```python
from build123d import *

# Parameters (mm, degrees)
SKETCH_1_R      = 50
SKETCH_1_R_2    = 40
EXTRUDE_1_DEPTH = 85
CHAMFER_1_SIZE  = 1
M10X1_0_1_D     = 9
M10X1_0_1_DEPTH = 25
M10X1_0_1_TIP   = 2.703872786


with BuildPart() as part:
    # 草图1 → 凸台-拉伸1 (new body)
    with BuildSketch(Plane(origin=(0, 0, 0), x_dir=(0, 0, -1), z_dir=(1, 0, 0))):
        Circle(SKETCH_1_R)
        Circle(SKETCH_1_R_2, mode=Mode.SUBTRACT)
    extrude(amount=EXTRUDE_1_DEPTH)

    # 倒角1
    chamfer_1_edges = [part.edges().sort_by_distance(p)[0] for p in [
        (0, 0, 50),
        (85, 0, 50),
        (0, 0, 40),
        (85, 0, 40),
    ]]
    chamfer(chamfer_1_edges, length=CHAMFER_1_SIZE)

    # M10x1.0 螺纹孔1
    with Locations(Plane(origin=(0, 50, 0), x_dir=(1, 0, 0), z_dir=(0, 1, 0))):
        with Locations((70, 0)):
            Hole(M10X1_0_1_D / 2, depth=M10X1_0_1_DEPTH)
            with Locations((0, 0, -(M10X1_0_1_DEPTH + M10X1_0_1_TIP / 2))):  # 118° drill point
                Cone(0, M10X1_0_1_D / 2, M10X1_0_1_TIP, mode=Mode.SUBTRACT)


solid = part.part
```
Could you check a few things on this model? Use its own coordinates, in mm. Coordinates: 2 decimals unless noted, no trailing zeros. Write each loop counter-clockwise with the first axis right and the second up, starting at its lowest first coordinate (ties: lowest second). Pieces come first, ordered by that corner, then holes. Notation, with made-up numbers: (64, 1) - (95, 1) arc R22 cw to (95, 15) - close; hole circle Ø6 at (38.25, 34.25). An arc over 180 degrees is marked (long way). Use a Markdown table: item, result.
Q1. Thinking about a two-plate mould opening in X: for faces 1 (the cylindrical face through (65.84, 44.8, 1.72)), 2 (the flat face through (85, -40, 11)), 3 (the flat face through (0, -40, 11)), which applies, +X half, -X half, draft (parallel to the pull), parting line (faces both ways), or undercut?
Geometry check:
| item | result |
|---|---|
| face 1 | undercut |
| face 2 | +X half |
| face 3 | -X half |
Q2. Imagine slicing it at A-A (z = 0). List the corners of the cut face in (x, y) for me.
Geometry check:
| item | result |
|---|---|
| outline | (0, -49) - (1, -50) - (84, -50) - (85, -49) - (85, -41) - (84, -40) - (1, -40) - (0, -41) - close; (0, 41) - (1, 40) - (65.5, 40) - (65.5, 50) - (1, 50) - (0, 49) - close; (74.5, 40) - (84, 40) - (85, 41) - (85, 49) - (84, 50) - (74.5, 50) - close |
Q3. I'm going to push flat-ended pins straight in: pin 1 Ø4 at (x, z) = (50, -2) entering from -Y; pin 2 Ø5 at (y, z) = (-7.5, 38) entering from +X; pin 3 Ø5 at (x, y) = (46, -23.5) entering from +Z; pin 4 Ø5 at (x, z) = (8.5, 34) entering from +Y. Where does each tip first touch, or does it pass through?
Geometry check:
| item | result |
|---|---|
| pin 1 | stops at y = -50 |
| pin 2 | stops at x = 85 |
| pin 3 | stops at z = 45.38 |
| pin 4 | stops at y = 38.83 |
Q4. Imagine slicing it at B-B (y = 0). List the corners of the cut face in (x, z) for me, and give its area (3 significant figures).
Geometry check:
| item | result |
|---|---|
| outline | (0, -49) - (1, -50) - (84, -50) - (85, -49) - (85, -41) - (84, -40) - (1, -40) - (0, -41) - close; (0, 41) - (1, 40) - (84, 40) - (85, 41) - (85, 49) - (84, 50) - (1, 50) - (0, 49) - close |
| area | 1,700 mm2 |
Q5. Please list where these lines run through material, in increasing order: L1, parallel to Y at x = 22, z = 0; L2, parallel to Y at x = 4, z = 33; L3, parallel to Z at x = 28, y = 31.
Geometry check:
| item | result |
|---|---|
| L1 | y = -50 to -40, 40 to 50 |
| L2 | y = -37.56 to -22.61, 22.61 to 37.56 |
| L3 | z = -39.23 to -25.28, 25.28 to 39.23 |
Q6. Imagine slicing it at C-C (x = 41). List the corners of the cut face in (y, z) for me.
Geometry check:
| item | result |
|---|---|
| outline | circle Ø100 at (0, 0); hole circle Ø80 at (0, 0) |
Q7. Imagine slicing it at D-D (x = 70). List the corners of the cut face in (y, z) for me.
Geometry check:
| item | result |
|---|---|
| outline | (39.75, -4.5) arc R40 cw (long way) to (39.75, 4.5) - (49.8, 4.5) arc R50 ccw (long way) to (49.8, -4.5) - close |
